Could you check a few things on this model? Use its own coordinates, in mm. A direction names the side the tool comes from. Give positions to 0.01 mm unless a question says otherwise; leave off trailing zeros. Order: outer loops, then holes, each group sorted by start corner. A loop starts at its lowest first (then second) coordinate and runs counter-clockwise, first axis right, second up. Notation, with made-up numbers: (61.25, -34.75) -> (74.25, -34.75) arc R33 ccw to (74.25, -3.75) -> close; hole circle Ø4 at (27.5, 42). An arc over 180 degrees is marked (long way). One line per item, written item: value.
```python
from build123d import *

# Parameters (mm, degrees)
F0_W     = 76.2
F0_H     = 12.7
F1_DEPTH = 25.4
F2_R     = 12.7
F3_DEPTH = 25.4
F4_DEPTH = 12.7
F5_R     = 6.35
F6_DEPTH = 38.1
F8_DEPTH = 12.7


with BuildPart() as f1:
    # F0 (on Front) → F1 (new body)
    with BuildSketch(Plane.XZ):
        with Locations((-9.585544682, 10.4771234242)):
            Rectangle(F0_W, F0_H)
    extrude(amount=F1_DEPTH)

    # F2 (on face) → F3 (join)
    with BuildSketch(Plane.XY.offset(16.8271234242)):
        with Locations((-34.985544682, -12.7)):
            Circle(F2_R)
    extrude(amount=F3_DEPTH)

    # F4 (cut): faces of the model
    f4_faces = [f1.faces().sort_by_distance(p)[0] for p in [
        (-44.8487718574, -2.8367728246, 16.8271234242),
        (-44.8487718574, -22.5632271754, 16.8271234242),
    ]]
    extrude(f4_faces, amount=-F4_DEPTH, mode=Mode.SUBTRACT)

    # F5 (on face) → F6 (cut)
    with BuildSketch(Plane.XY.offset(42.2271234242)):
        with Locations((-34.985544682, -12.7)):
            Circle(F5_R)
    extrude(amount=-F6_DEPTH, mode=Mode.SUBTRACT)

    # F7 (on face) → F8 (cut)
    with BuildSketch(Plane.XY.offset(16.8271234242)):
        with BuildLine():
            ThreePointArc((-9.585544682, -19.05), (-5.0954166214, -17.1901280605), (-3.235544682, -12.7))
            ThreePointArc((-3.235544682, -12.7), (-5.0954166214, -8.2098719395), (-9.585544682, -6.35))
            ThreePointArc((-9.585544682, -6.35), (-15.935544682, -12.7), (-9.585544682, -19.05))
        make_face()
        with BuildLine():
            ThreePointArc((-9.585544682, -6.35), (-5.0954166214, -8.2098719395), (-3.235544682, -12.7))
            ThreePointArc((-3.235544682, -12.7), (-5.0954166214, -17.1901280605), (-9.585544682, -19.05))
            Line((-9.585544682, -19.05), (15.814455318, -19.05))
            ThreePointArc((15.814455318, -19.05), (9.464455318, -12.7), (15.814455318, -6.35))
            Line((15.814455318, -6.35), (-9.585544682, -6.35))
        make_face()
        with BuildLine():
            ThreePointArc((22.164455318, -12.7), (20.3045833786, -8.2098719395), (15.814455318, -6.35))
            ThreePointArc((15.814455318, -6.35), (9.464455318, -12.7), (15.814455318, -19.05))
            ThreePointArc((15.814455318, -19.05), (20.3045833786, -17.1901280605), (22.164455318, -12.7))
        make_face()
        with BuildLine():
            ThreePointArc((15.814455318, 0), (27.816257265, -12.7), (15.814455318, -25.4))
            Line((15.814455318, -25.4), (28.514455318, -25.4))
            Line((28.514455318, -25.4), (28.514455318, 0))
            Line((28.514455318, 0), (15.814455318, 0))
        make_face()
    extrude(amount=-F8_DEPTH, mode=Mode.SUBTRACT)


solid = f1.part
```
1) Suppose I cut it at C-C, the plane y = -8.75. Write out the boundary of the cut face in (x, z), then the cut area to 3 significant figures.
Answer below:
outline: (-47.06, 4.13) -> (-39.96, 4.13) -> (-39.96, 42.23) -> (-47.06, 42.23) -> close; (-30.01, 4.13) -> (-14.56, 4.13) -> (-14.56, 16.83) -> (-22.92, 16.83) -> (-22.92, 42.23) -> (-30.01, 42.23) -> close; (20.79, 4.13) -> (27.19, 4.13) -> (27.19, 16.83) -> (20.79, 16.83) -> close
area: 728 mm2
2) We'd pull the mould along Y, two halves only. Please class faces 1 (the cylindrical face through (-36.36, -18.9, 23.44)), 2 (the cylindrical face through (-15.934, -12.56, 10.566)), 3 (the flat face through (-10, 0, 11)), 4 (the flat face through (-19, -13, 4.127)): +Y half, -Y half, draft (parallel to the pull), parting line (faces both ways), or undercut.
Answer below:
face 1: undercut
face 2: undercut
face 3: +Y half
face 4: draft
3) Suppose I cut it at D-D, the plane z = 26.5. Write out the boundary of the cut face in (x, y).
Answer below:
outline: circle Ø25.4 at (-34.99, -12.7); hole circle Ø12.7 at (-34.99, -12.7)
4) Suppose I cut it at B-B, the plane x = -37. Write out the boundary of the cut face in (y, z), then the cut area to 3 significant figures.
Answer below:
outline: (-25.24, 4.13) -> (-18.72, 4.13) -> (-18.72, 42.23) -> (-25.24, 42.23) -> close; (-6.68, 4.13) -> (-0.16, 4.13) -> (-0.16, 42.23) -> (-6.68, 42.23) -> close
area: 497 mm2
5) For faces 5 (the cylindrical face through (-47.673, -12.142, 27.144)), 6 (the cylindrical face through (27.813, -12.43, 10.566)), 7 (the flat face through (3, -19.05, 11)), which set-ups out of +Z, -Z, +X, -X, +Y, -Y let a thin tool reach every point of the face, with its end or its side?
Answer below:
face 5: +Z
face 6: +Z, -Z, +X
face 7: +Z, -Z
6) If I drill on line 1 along Y through (x, z) = (-7, 14.5); line 2 along Z through (x, y) = (-10, -21); line 3 along Y through (x, z) = (21.5, 10.5), over which ranges is the centre line in solid material (lowest first)?
Answer below:
line 1: y = -25.4 to -19.05, -6.35 to 0
line 2: z = 4.13 to 16.83
line 3: y = -23.69 to -15.53, -9.87 to -1.71
7) Suppose I cut it at A-A, the plane z = 12. Write out the boundary of the cut face in (x, y), then the cut area to 3 significant figures.
Answer below:
outline: (-34.99, -25.4) -> (15.81, -25.4) arc R12.72 ccw to (15.81, 0) -> (-34.99, 0) arc R12.7 ccw to start; hole circle Ø12.7 at (-34.99, -12.7); hole (-9.59, -19.05) -> (15.81, -19.05) arc R6.35 ccw to (15.81, -6.35) -> (-9.59, -6.35) arc R6.35 ccw to start
area: 1,200 mm2
8) For P1, Ø5, axis at x = -6.5, y = -10, coming from the -Z side; P2, Ø8, axis at x = 10, y = -3.5, coming from the +Z side; P3, Ø8, axis at y = -22.5, z = 30.5, coming from the -X side; P4, Ø1, axis at y = -19.5, z = 28.5, coming from the -X side, each with a flat end and sliding along its axis, tell me the tip position at first contact or that it passes through.
Answer below:
P1: passes through
P2: stops at z = 16.83
P3: stops at x = -46.28
P4: stops at x = -46.01
